```python
from build123d import *

# Parameters (mm, degrees)
BOSS_EXTRU_1_DEPTH = 3
SKETCH1_R          = 2
CUT_EXTRUDE1_DEPTH = 37.557629685


with BuildPart() as part:
    # Esquisse1 → Boss.-Extru.1 (new body)
    with BuildSketch(Plane.XY):
        with BuildLine():
            Line((-1.901457503, 12), (-34.401457503, 0))
            Line((-34.401457503, 0), (-21.901457503, -12))
            Line((-21.901457503, -12), (23.598542497, -12))
            add(Edge.make_bspline(
                [(23.598542497, -12), (27.098542497, -12), (28.848542497, -10.25), (30.598542497, -8.5)],
                knots=[0, 0, 0, 0, 0.5, 0.5, 0.5, 0.5], degree=3))
            Line((30.598542497, -8.5), (30.598542497, 8.5))
            add(Edge.make_bspline(
                [(23.598542497, 12), (27.098542497, 12), (28.848542497, 10.25), (30.598542497, 8.5)],
                knots=[0, 0, 0, 0, 0.5, 0.5, 0.5, 0.5], degree=3))
            Line((23.598542497, 12), (-1.901457503, 12))
        make_face()
        Polygon((-2.401457503, 2), (-2.401457503, 6), (20.598542497, 6), (20.598542497, 2), (25.598542497, 2), (25.598542497, -2), (20.598542497, -2), (20.598542497, -6), (-2.401457503, -6), (-2.401457503, -2), (-7.401457503, -2), (-7.401457503, 2), align=None, mode=Mode.SUBTRACT)
    extrude(amount=BOSS_EXTRU_1_DEPTH)

    # Sketch1 → Cut-Extrude1 (cut, through all)
    with BuildSketch(Plane.XY.offset(3)):
        with Locations((-20.901457503, 0)):
            Circle(SKETCH1_R)
    extrude(amount=-CUT_EXTRUDE1_DEPTH, mode=Mode.SUBTRACT)


solid = part.part
```
Design review of the part built by this model. Coordinates are the model's own, in mm. A direction names the side the tool comes from. Round coordinates to 2 decimals unless told otherwise and drop trailing zeros. Write each loop counter-clockwise with the first axis right and the second up, starting at its lowest first coordinate (ties: lowest second). Pieces come first, ordered by that corner, then holes.
Item 1: We need section B-B on y = 5.25. Write out the cut boundary in (x, z), and give its area (3 significant figures).
Item 2: For faces 1 (the flat face through (-2, -8, 3)), 2 (the flat face through (-2.401, -4, 1)), list the 3-axis set-ups (+Z, -Z, +X, -X, +Y, -Y) from which the entire face can be reached by the end or side of a thin tool; tool diameter is ignored.
Item 3: We need section A-A on x = 12. Write out the cut boundary in (y, z), and give its area (3 significant figures).
Item 4: We need section C-C on z = 2. State how many separate pieces and enclosed holes the cut face has, and give its area (3 significant figures).
Item 5: Clearance check with flat-ended pins moving along their axes: pin 1 Ø1.5 at (y, z) = (0, 1.5) entering from -X; pin 2 Ø1.5 at (x, z) = (-26.5, 1.5) entering from +Y; pin 3 Ø3.5 at (x, y) = (-20.9, 0) entering from -Z. State where each tip first meets the part, or that it passes through.
Item 6: We need section D-D on x = -13. Write out the cut boundary in (y, z).
Item 7: For probe 1 along Y at (x, z) = (23.5, 2.1); probe 2 along Y at (x, z) = (20, 1.85); probe 3 along X at (y, z) = (-1, 1.25), list the stretches that pass through material, from the lowest coordinate up.
Item 8: The part is to be moulded in two halves that separate along X. For faces 3 (the flat face through (30.599, 0, 1)), 4 (the flat face through (-5, -2, 1)), 5 (the flat face through (11, 12, 1)), 6 (the flat face through (-17.924, 6.084, 1.479)), say which applies: +X half, -X half, draft (parallel to the pull), parting line (faces both ways), or undercut.
Returned:
1. outline: (-20.18, 0) - (-2.4, 0) - (-2.4, 3) - (-20.18, 3) - close; (20.6, 0) - (30.6, 0) - (30.6, 3) - (20.6, 3) - close
1. area: 83.3 mm2
2. face 1: +Z, +X, -X, +Y, -Y
2. face 2: +Z, -Z
3. outline: (-12, 0) - (-6, 0) - (-6, 3) - (-12, 3) - close; (6, 0) - (12, 0) - (12, 3) - (6, 3) - close
3. area: 36.0 mm2
4. separate pieces: 1
4. enclosed holes: 2
4. area: 946 mm2
5. pin 1: stops at x = -34.4
5. pin 2: stops at y = 3.19
5. pin 3: passes through
6. outline: (-12, 0) - (7.9, 0) - (7.9, 3) - (-12, 3) - close
7. probe 1: y = -12 to -2, 2 to 12
7. probe 2: y = -12 to -6, 6 to 12
7. probe 3: x = -33.36 to -22.63, -19.17 to -7.4, 25.6 to 30.6
8. face 3: +X half
8. face 4: undercut
8. face 5: draft
8. face 6: -X half
